```python
from build123d import *

# Parameters (mm, degrees)
SKETCH_1_W               = 102
SKETCH_1_H               = 64
SKETCH_1_W_2             = 100
SKETCH_1_H_2             = 62
EXTRUDE_1_DEPTH          = 50
SKETCH_1_3_R             = 1.5
EXTRUDE_2_DEPTH          = 9.72
SKETCH_4_W               = 102
SKETCH_4_H               = 1
EXTRUDE_3_DEPTH          = 64
SKETCH_1_5_W             = 76
SKETCH_1_5_H             = 25.8
CUT_EXTRUDE_1_DEPTH      = 1
CUT_EXTRUDE_2_DEPTH      = 102
CUT_EXTRUDE_2_DEPTH_BACK = 1
SKETCH_5_R               = 1
SKETCH_6_R               = 1.25
SKETCH_6_W               = 6
SKETCH_6_H               = 6
CUT_EXTRUDE_3_DEPTH      = 10


with BuildPart() as part:
    # Sketch 1 → Extrude 1 (new body)
    with BuildSketch(Plane.XY):
        with Locations((53, 34)):
            Rectangle(SKETCH_1_W, SKETCH_1_H)
        with Locations((53, 34)):
            Rectangle(SKETCH_1_W_2, SKETCH_1_H_2, mode=Mode.SUBTRACT)
    extrude(amount=EXTRUDE_1_DEPTH)

    # Sketch 1_3 → Extrude 2 (add)
    # profile 1 of 4: a face of its own
    with BuildSketch(Plane.XY):
        with BuildLine():
            Line((6.5, 65), (3, 65))
            Line((3, 65), (3, 61.5))
            Line((3, 61.5), (4, 61.5))
            ThreePointArc((4, 61.5), (8.267766953, 59.732233047), (6.5, 64))
            Line((6.5, 64), (6.5, 65))
        make_face()
        with Locations((6.5, 61.5)):
            Circle(SKETCH_1_3_R, mode=Mode.SUBTRACT)
    # profile 2 of 4: a face of its own
    with BuildSketch(Plane.XY):
        with BuildLine():
            Line((103, 65), (99.5, 65))
            Line((99.5, 65), (99.5, 64))
            ThreePointArc((99.5, 64), (97.732233047, 59.732233047), (102, 61.5))
            Line((102, 61.5), (103, 61.5))
            Line((103, 61.5), (103, 65))
        make_face()
        with Locations((99.5, 61.5)):
            Circle(SKETCH_1_3_R, mode=Mode.SUBTRACT)
    # profile 3 of 4: a face of its own
    with BuildSketch(Plane.XY):
        with BuildLine():
            Line((103, 3), (103, 6.5))
            Line((103, 6.5), (102, 6.5))
            ThreePointArc((102, 6.5), (97.732233047, 8.267766953), (99.5, 4))
            Line((99.5, 4), (99.5, 3))
            Line((99.5, 3), (103, 3))
        make_face()
        with Locations((99.5, 6.5)):
            Circle(SKETCH_1_3_R, mode=Mode.SUBTRACT)
    # profile 4 of 4: a face of its own
    with BuildSketch(Plane.XY):
        with BuildLine():
            Line((4, 6.5), (3, 6.5))
            Line((3, 6.5), (3, 3))
            Line((3, 3), (6.5, 3))
            Line((6.5, 3), (6.5, 4))
            ThreePointArc((6.5, 4), (8.267766953, 8.267766953), (4, 6.5))
        make_face()
        with Locations((6.5, 6.5)):
            Circle(SKETCH_1_3_R, mode=Mode.SUBTRACT)
    extrude(amount=EXTRUDE_2_DEPTH)

    # Sketch 4 → Extrude 3 (add)
    with BuildSketch(Plane(origin=(0, 66, 0), x_dir=(1, 0, 0), z_dir=(0, 1, 0))):
        with Locations((53, 0.5)):
            Rectangle(SKETCH_4_W, SKETCH_4_H)
    extrude(amount=-EXTRUDE_3_DEPTH)

    # Sketch 1_5 → Cut-Extrude 1 (cut)
    with BuildSketch(Plane.XY):
        with Locations((53, 34)):
            Rectangle(SKETCH_1_5_W, SKETCH_1_5_H)
    extrude(amount=-CUT_EXTRUDE_1_DEPTH, mode=Mode.SUBTRACT)

    # Sketch 5 → Cut-Extrude 2 (cut, two sides: drawn at the far end of the back side and taken through both)
    with BuildSketch(Plane.ZY.offset(-103).offset(-CUT_EXTRUDE_2_DEPTH_BACK)):
        with Locations(Location((43.5, 7.5, 0), (0, 0, 90))):
            Circle(SKETCH_5_R)
        with Locations(Location((43.5, 60.5, 0), (0, 0, 90))):
            Circle(SKETCH_5_R)
    extrude(amount=CUT_EXTRUDE_2_DEPTH + CUT_EXTRUDE_2_DEPTH_BACK, mode=Mode.SUBTRACT)

    # Sketch 6 → Cut-Extrude 3 (cut)
    with BuildSketch(Plane(origin=(0, 66, 0), x_dir=(1, 0, 0), z_dir=(0, 1, 0))):
        with Locations(Location((27, -27, 0), (0, 0, 180))):
            Circle(SKETCH_6_R)
        with Locations(Location((38, -27, 0), (0, 0, 180))):
            Circle(SKETCH_6_R)
        with Locations(Location((53, -27, 0), (0, 0, 180))):
            Circle(SKETCH_6_R)
        with Locations(Location((64, -27, 0), (0, 0, 180))):
            Circle(SKETCH_6_R)
        with Locations((32.5, -30.5)):
            Rectangle(SKETCH_6_W, SKETCH_6_H)
        with Locations((58.5, -30.5)):
            Rectangle(SKETCH_6_W, SKETCH_6_H)
    extrude(amount=-CUT_EXTRUDE_3_DEPTH, mode=Mode.SUBTRACT)


solid = part.part
```
CAD build for the part. Positions are in the model's coordinates, mm. A direction names the side the tool comes from. Give positions to 0.01 mm unless a question says otherwise; leave off trailing zeros. Loops run counter-clockwise (first coordinate to the right, second up) from the corner with the lowest first, then second, coordinate; pieces in that order, holes last. Notation, with made-up numbers: M -23,5 L 15,5 A15 ccw 15,32 Z; hole C -3,3 d10. An arc over 180 degrees is marked long. Use one line per item in the form item = value.
Item 1: Slice it at C-C (x = 27). List the corners of the cut face in (y, z).
Determined:
outline = M 2,-1 L 21.1,-1 L 21.1,0 L 3,0 L 3,50 L 2,50 Z; M 46.9,-1 L 66,-1 L 66,25.75 L 65,25.75 L 65,0 L 46.9,0 Z; M 65,28.25 L 66,28.25 L 66,50 L 65,50 Z
Item 2: Which spindle directions (+Z, -Z, +X, -X, +Y, -Y) get a long thin tool onto all of the face, cutting with end or side? Do faces 1 (the face through (103, 34, 25)), 2 (the face through (25.845, 65.507, 26.521)). Say none if no direction does.
Determined:
face_1 = +Z
face_2 = +Y
Item 3: Slice it at B-B (z = 4). List the corners of the cut face in (x, y).
Determined:
outline = M 2,2 L 104,2 L 104,66 L 2,66 Z; hole M 3,6.5 L 4,6.5 A2.5 cw long 6.5,4 L 6.5,3 L 99.5,3 L 99.5,4 A2.5 cw long 102,6.5 L 103,6.5 L 103,61.5 L 102,61.5 A2.5 cw long 99.5,64 L 99.5,65 L 6.5,65 L 6.5,64 A2.5 cw long 4,61.5 L 3,61.5 Z; hole C 6.5,6.5 d3; hole C 6.5,61.5 d3; hole C 99.5,6.5 d3; hole C 99.5,61.5 d3
Item 4: Slice it at D-D (z = 29.5). List the corners of the cut face in (x, y).
Determined:
outline = M 2,2 L 104,2 L 104,66 L 61.5,66 L 61.5,65 L 103,65 L 103,3 L 3,3 L 3,65 L 29.5,65 L 29.5,66 L 2,66 Z; M 35.5,65 L 55.5,65 L 55.5,66 L 35.5,66 Z
Item 5: Flat gauge pins, fed straight in: pin 1 (1.5 mm diameter, centred on x = 99, y = 61, fed in from +Z); pin 2 (1.8 mm diameter, centred on y = 7.5, z = 43.5, fed in from +X); pin 3 (1.8 mm diameter, centred on x = 5, y = 61, fed in from +Z). Where does each tip first touch, or does it go through?
Determined:
pin_1 = 0
pin_2 = through
pin_3 = 9.72
Item 6: Slice it at A-A (y = 36.5). List the corners of the cut face in (x, z), plus the area to 3 significant figures.
Determined:
outline = M 2,-1 L 15,-1 L 15,0 L 3,0 L 3,50 L 2,50 Z; M 91,-1 L 104,-1 L 104,50 L 103,50 L 103,0 L 91,0 Z
area = 126 mm2
Item 7: Two-plate mould, pull along Y, no slides. Class faces 3 (the face through (52, 20, -1)), 4 (the face through (2.507, 59.763, 42.824)): pulls with the +Y half, pulls with the -Y half, needs draft (parallel to the pull), parting line crosses it, or undercut.
Determined:
face_3 = needs draft
face_4 = undercut
Item 8: Drill centre lines: probe 1 along Y at (x, z) = (2.3, 43.5); probe 2 along X at (y, z) = (23, 44); probe 3 along Y at (x, z) = (94, 11). Where is each one in solid material? Low to high. Write a range as from..to.
Determined:
probe_1 = 2..6.5, 8.5..59.5, 61.5..66
probe_2 = 2..3, 103..104
probe_3 = 2..3, 65..66
